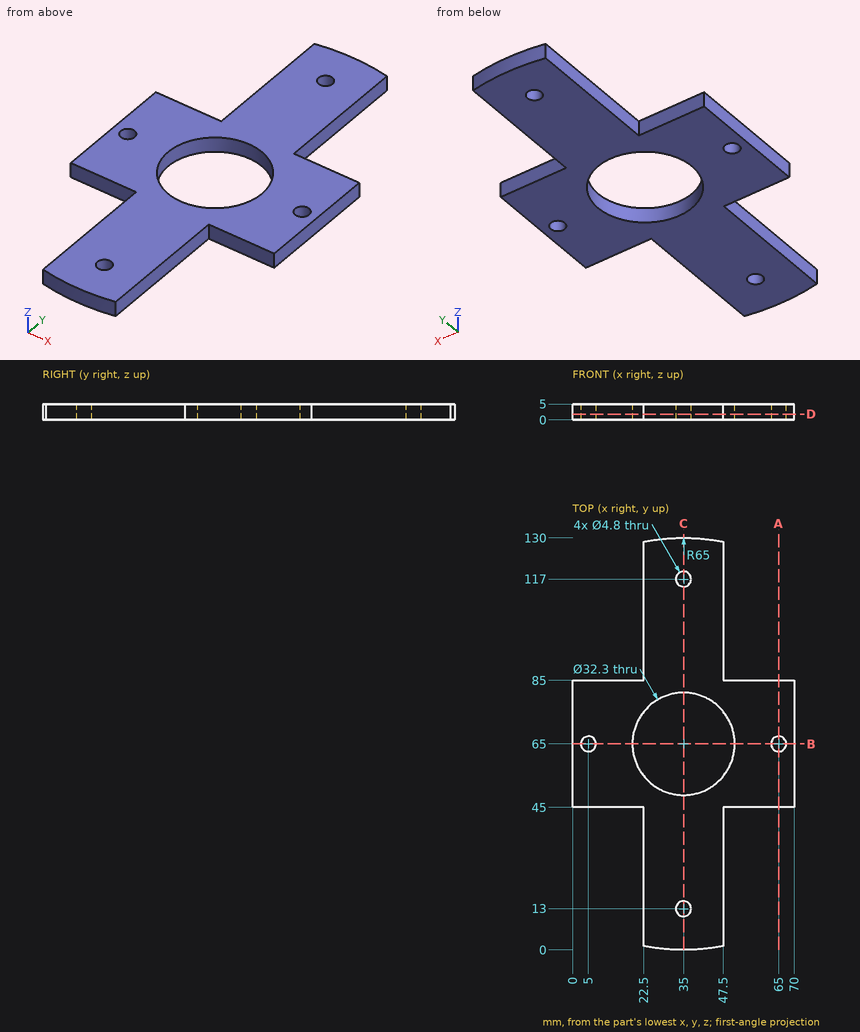
Verification items for this drawing (mm, ordinates from the low corner). Coordinates: 2 decimals unless noted, no trailing zeros. Order: outer loops, then holes, each group sorted by start corner. A loop starts at its lowest first (then second) coordinate and runs counter-clockwise, first axis right, second up. Notation, with made-up numbers: M 30,-39.75 L 78,-39.75 A22 cw 78,-4.75 Z; hole C -6.75,-27 d3. An arc over 180 degrees is marked long. One line per item, written item: value. Start each with the question number.
Item 1: Sectioned sample at A-A on x = 65. Record the cut outline in (y, z), then the cut area to 3 significant figures.
Item 2: Depth check by flat-ended pin: P1, Ø1, axis at x = 8, z = 2.5, coming from the -Y side; P2, Ø1.5, axis at x = 61, z = 1.5, coming from the +Y side. Enter the tip coordinate at first touch or a pass-through.
Item 3: Sectioned sample at C-C on x = 35. Record the cut outline in (y, z).
Item 4: Sectioned sample at D-D on z = 1.8. Record the cut outline in (x, y).
Item 5: Thickness scan on probe 1 along Y at (x, z) = (35, 3.7); probe 2 along Y at (x, z) = (37, 1.55); probe 3 along X at (y, z) = (17, 3.95). Record the ranges inside material, lowest first.
Item 6: Sectioned sample at B-B on y = 65. Record the cut outline in (x, z), then the cut area to 4 significant figures.
Calculated:
1. outline: M 45,0 L 62.6,0 L 62.6,5 L 45,5 Z; M 67.4,0 L 85,0 L 85,5 L 67.4,5 Z
1. area: 176 mm^2
2. P1: y = 45
2. P2: y = 85
3. outline: M 0,0 L 10.6,0 L 10.6,5 L 0,5 Z; M 15.4,0 L 48.85,0 L 48.85,5 L 15.4,5 Z; M 81.15,0 L 114.6,0 L 114.6,5 L 81.15,5 Z; M 119.4,0 L 130,0 L 130,5 L 119.4,5 Z
4. outline: M 0,45 L 22.5,45 L 22.5,1.21 A65 ccw 47.5,1.21 L 47.5,45 L 70,45 L 70,85 L 47.5,85 L 47.5,128.79 A65 ccw 22.5,128.79 L 22.5,85 L 0,85 Z; hole C 5,65 d4.8; hole C 35,65 d32.3; hole C 35,13 d4.8; hole C 35,117 d4.8; hole C 65,65 d4.8
5. probe 1: 0 to 10.6, 15.4 to 48.85, 81.15 to 114.6, 119.4 to 130
5. probe 2: 0.03 to 11.67, 14.33 to 48.97, 81.03 to 115.67, 118.33 to 129.97
5. probe 3: 22.5 to 47.5
6. outline: M 0,0 L 2.6,0 L 2.6,5 L 0,5 Z; M 7.4,0 L 18.85,0 L 18.85,5 L 7.4,5 Z; M 51.15,0 L 62.6,0 L 62.6,5 L 51.15,5 Z; M 67.4,0 L 70,0 L 70,5 L 67.4,5 Z
6. area: 140.5 mm^2
